Autodesk Inventor part; units mm, degrees
ref_plane "YZ Plane" through (0, 0, 0) normal (1, 0, 0) x (0, 1, 0)
ref_plane "XZ Plane" through (0, 0, 0) normal (0, 1, 0) x (-1, 0, 0)
ref_plane "XY Plane" through (0, 0, 0) normal (0, 0, 1) x (1, 0, 0)
sketch "Sketch1" plane through (0, 0, 0) normal (0, 0, 1) x (1, 0, 0)
  line L0 (44.7404, -16.6127) -> (-43.4425, -16.6127)
  arc A0 (44.7404, -16.6127) -> (46.8806, -2.4194) centre (44.7404, -9.3547) ccw
  arc A1 (-41.9354, -2.4194) -> (-43.4425, -16.6127) centre (-44.2086, -9.3547) ccw
  line L1 (48.387, 82.2579) -> (48.387, 9.6774)
  arc A2 (-25.6909, 70.9206) -> (-41.9354, 70.9676) centre (-33.8226, 67.6679) ccw
  line L2 (-41.9354, -2.4194) -> (-41.9354, 70.9676)
  line L3 (-25.6909, -2.4194) -> (-25.6909, 70.9206)
  line L4 (-25.6909, -2.4194) -> (46.8806, -2.4194)
  line L5 (-57.912, 100.584) -> (69.088, 100.584)
  line L6 (69.088, 100.584) -> (69.088, -26.416)
  line L7 (69.088, -26.416) -> (-57.912, -26.416)
  line L8 (-57.912, -26.416) -> (-57.912, 100.584)
  arc A3 (32.258, 9.6774) -> (48.387, 9.6774) centre (40.3225, 12.3185) ccw
  arc A4 (48.387, 82.2579) -> (48.387, 96.774) centre (42.691, 89.5159) ccw
  line L9 (32.258, 82.2579) -> (-41.9354, 82.2579)
  line L10 (48.387, 96.774) -> (-41.9354, 96.774)
  line L11 (32.258, 9.6774) -> (32.258, 82.2579)
  arc A5 (-41.9354, 96.774) -> (-41.9354, 82.2579) centre (-43.9372, 89.5159) ccw
  point P0 (0, 0)
  dimension "d0" = 127
  dimension "d1" = 127
extrude "Extrusion1" add sketch "Sketch1" along normal blind 12.7
sketch "Sketch2" plane through (0, 0, 12.7) normal (0, 0, 1) x (1, 0, 0)
  circle A0 centre (22, 7) radius 6.35
  circle A1 centre (-16, 6.6796) radius 6.35
  circle A2 centre (-16, 72) radius 6.35
  circle A3 centre (22, 72) radius 6.35
  point P0 (0, 0)
  dimension "d4" = 12.7
  dimension "d5" = 12.7
  dimension "d6" = 12.7
  dimension "d7" = 12.7
hole "Hole1" at (-16, 6.6796, 12.7) at (22, 72, 12.7) at (-16, 72, 12.7) at (22, 7, 12.7) direction (0, 0, -1) diameter 12.7 end through all
sketch "Sketch3" plane through (0, 0, 12.7) normal (0, 0, 1) x (1, 0, 0)
  arc A0 (20.8111, 55.9606) -> (21.1932, 22.4134) centre (4.585, 39) ccw
  arc A1 (8, 45) -> (8.4788, 33.299) centre (4.585, 39) ccw
  arc A2 (6.7211, 45.565) -> (19.6498, 57) centre (12.644, 51.8946) ccw
  arc A3 (18.8086, 20.3282) -> (5.9993, 32.2426) centre (13.4301, 27.3887) ccw
  circle A4 centre (-16, 72) radius 6.35
  circle A5 centre (-16, 6.6796) radius 6.35
  circle A6 centre (22, 72) radius 6.35
  circle A7 centre (22, 7) radius 6.35
  arc A8 (48.387, 82.2579) -> (48.387, 96.774) centre (42.691, 89.5159) ccw
  line L0 (48.387, 82.2579) -> (48.387, 9.6774)
  arc A9 (32.258, 9.6774) -> (48.387, 9.6774) centre (40.3225, 12.3185) ccw
  line L1 (32.258, 9.6774) -> (32.258, 82.2579)
  line L2 (32.258, 82.2579) -> (-41.9354, 82.2579)
  arc A10 (-41.9354, 96.774) -> (-41.9354, 82.2579) centre (-43.9372, 89.5159) ccw
  line L3 (-41.9354, 96.774) -> (48.387, 96.774)
  arc A11 (-41.9354, -2.4194) -> (-43.4425, -16.6127) centre (-44.2086, -9.3547) ccw
  line L4 (-41.9354, -2.4194) -> (-41.9354, 70.9676)
  arc A12 (-25.6909, 70.9206) -> (-41.9354, 70.9676) centre (-33.8226, 67.6679) ccw
  line L5 (-25.6909, 70.9206) -> (-25.6909, -2.4194)
  line L6 (-25.6909, -2.4194) -> (46.8806, -2.4194)
  arc A13 (44.7404, -16.6127) -> (46.8806, -2.4194) centre (44.7404, -9.3547) ccw
  line L7 (44.7404, -16.6127) -> (-43.4425, -16.6127)
  line L8 (69.088, 100.584) -> (-57.912, 100.584)
  line L9 (-57.912, 100.584) -> (-57.912, -26.416)
  line L10 (-57.912, -26.416) -> (69.088, -26.416)
  line L11 (69.088, -26.416) -> (69.088, 100.584)
  point P0 (0, 0)
  point P1 (20.2164, 21.4898)
  point P2 (20.9887, 55.7889)
emboss "Emboss1" sketch "Sketch3" operation cut depth 12.7 direction (0, 0, -1) contours A2 A1 A3 A0
properties part number "newnameC" material "Polyethylene, High Density"
The model under review builds one solid part; all positions refer to its coordinate system, in mm. A direction names the side the tool comes from. Coordinates: 2 decimals unless noted, no trailing zeros. Write each loop counter-clockwise with the first axis right and the second up, starting at its lowest first coordinate (ties: lowest second). Pieces come first, ordered by that corner, then holes.
1) To check wall thickness, follow probe 1 along X at (y, z) = (41, 8); probe 2 along X at (y, z) = (72, 2.5); probe 3 along Y at (x, z) = (-16, 5.5). State the ranges of each line that lie inside material, in increasing order.
2) Machinability: for faces 1 (the face through (5, 38, 0)), 2 (the face through (48.387, 46, 6)), which of the approach directions +Z, -Z, +X, -X, +Y, -Y give a long, thin tool a straight path to every point of the face, cutting with its end or side? Answer none if there is none.
3) We need section C-C on x = -50. State the section outline as (y, z) points.
4) We need section A-A on x = -16. State the section outline as (y, z) points, then the cut area to 3 significant figures.
5) The part is to be moulded in two halves that separate along X. For faces 3 (the face through (-51.464, 89.322, 6.261)), 4 (the face through (-57.912, 36, 6)), 5 (the face through (5, 38, 12.7)), say which applies: pulls with the +X half, pulls with the -X half, needs draft (parallel to the pull), parting line crosses it, or undercut.
6) Clearance check with a flat-ended pin moving along its axis: pin 1 Ø19 at (x, y) = (-44.21, -9.35) entering from -Z. State where the tip first meets the part, or that it passes through.
7) We need section D-D on y = -10.5. State the section outline as (x, z) points.
8) We need section B-B on y = 7. State the section outline as (x, z) points (3 decimals), then the cut area to 3 significant figures.
Answer list:
1. probe 1: x = -57.91 to -41.94, -25.69 to -18.8, -2.02 to 32.26, 48.39 to 69.09
1. probe 2: x = -57.91 to -41.43, -26.21 to -22.35, -9.65 to 15.65, 28.35 to 32.26, 48.39 to 69.09
1. probe 3: y = -26.42 to -16.61, -2.42 to 0.33, 13.03 to 27.72, 50.28 to 65.65, 78.35 to 82.26, 96.77 to 100.58
2. face 1: -Z, +X, -X, +Y, -Y
2. face 2: +Z, -Z
3. outline: (-26.42, 0) - (-13.8, 0) - (-13.8, 12.7) - (-26.42, 12.7) - close; (-4.91, 0) - (85.05, 0) - (85.05, 12.7) - (-4.91, 12.7) - close; (93.98, 0) - (100.58, 0) - (100.58, 12.7) - (93.98, 12.7) - close
4. outline: (-26.42, 0) - (-16.61, 0) - (-16.61, 12.7) - (-26.42, 12.7) - close; (-2.42, 0) - (0.33, 0) - (0.33, 12.7) - (-2.42, 12.7) - close; (13.03, 0) - (27.72, 0) - (27.72, 12.7) - (13.03, 12.7) - close; (50.28, 0) - (65.65, 0) - (65.65, 12.7) - (50.28, 12.7) - close; (78.35, 0) - (82.26, 0) - (82.26, 12.7) - (78.35, 12.7) - close; (96.77, 0) - (100.58, 0) - (100.58, 12.7) - (96.77, 12.7) - close
4. area: 639 mm2
5. face 3: undercut
5. face 4: pulls with the -X half
5. face 5: needs draft
6. pin 1: stops at z = 0
7. outline: (-57.91, 0) - (-51.42, 0) - (-51.42, 12.7) - (-57.91, 12.7) - close; (51.91, 0) - (69.09, 0) - (69.09, 12.7) - (51.91, 12.7) - close
8. outline: (-57.912, 0) - (-41.935, 0) - (-41.935, 12.7) - (-57.912, 12.7) - close; (-25.691, 0) - (-22.342, 0) - (-22.342, 12.7) - (-25.691, 12.7) - close; (-9.658, 0) - (15.65, 0) - (15.65, 12.7) - (-9.658, 12.7) - close; (28.35, 0) - (33.71, 0) - (33.71, 12.7) - (28.35, 12.7) - close; (46.935, 0) - (69.088, 0) - (69.088, 12.7) - (46.935, 12.7) - close
8. area: 916 mm2
